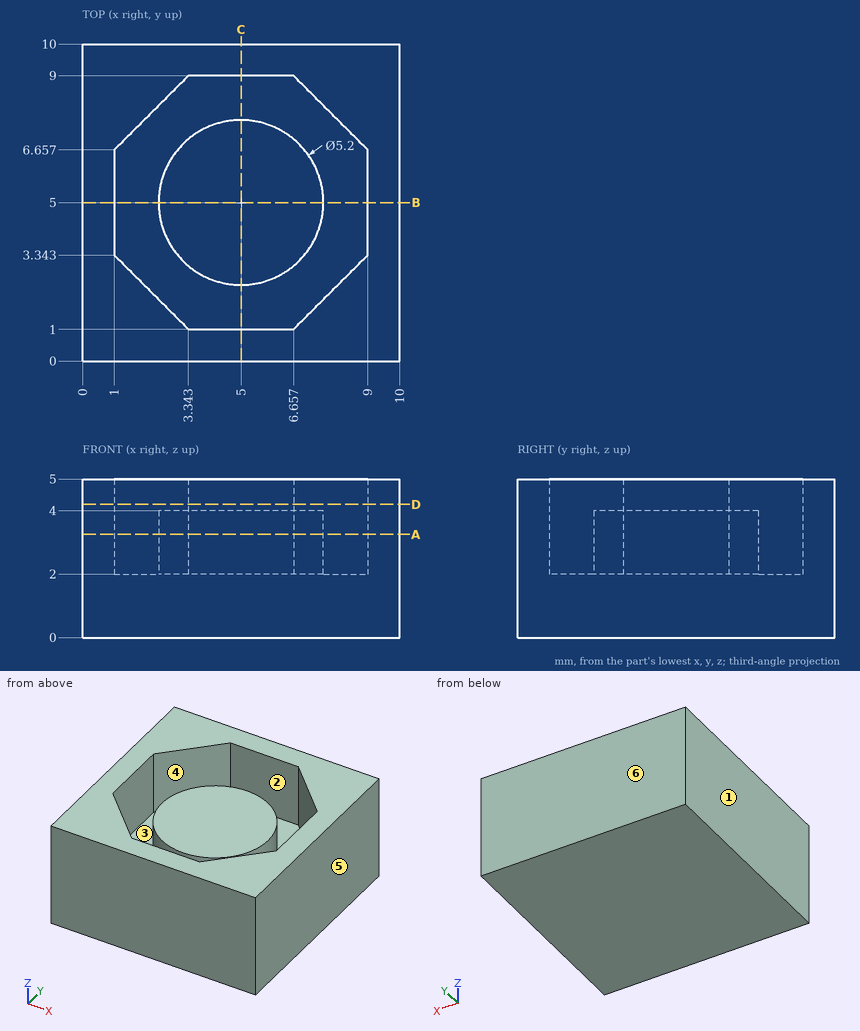
Answer from the drawing. Dimensions are ordinates in mm from the lowest x, y and z of the part. A direction names the side the tool comes from. Coordinates: 2 decimals unless noted, no trailing zeros. Loops run counter-clockwise (first coordinate to the right, second up) from the corner with the lowest first, then second, coordinate; pieces in that order, holes last. Notation, with made-up numbers: (87.5, 31) - (143.5, 31) arc R14 ccw to (143.5, 41) - close; hole circle Ø9 at (6, 13). An arc over 180 degrees is marked (long way). Use a Markdown table: item, result.
Item 1: Consider probe 1 along Y at (x, z) = (4, 2.1); probe 2 along Y at (x, z) = (6.25, 2.7); probe 3 along Y at (x, z) = (4, 4.4). Determine where each line is inside the solid, lowest interval first. Write a range as from..to.
Evaluation:
| item | result |
|---|---|
| probe 1 | y = 0..1, 2.6..7.4, 9..10 |
| probe 2 | y = 0..1, 2.72..7.28, 9..10 |
| probe 3 | y = 0..1, 9..10 |
Item 2: For the marked faces 1 and 2, determine the directions among +Z, -Z, +X, -X, +Y, -Y from which every point of the face is accessible in a straight line to the end or side of a thin tool.
Evaluation:
| item | result |
|---|---|
| face 1 | +Z, -Z, -X, +Y, -Y |
| face 2 | +Z |
Item 3: The mould has two halves that part along X. Classify the marked faces 3, 4, 5 and 6: +X half, -X half, draft (parallel to the pull), parting line (faces both ways), or undercut.
Evaluation:
| item | result |
|---|---|
| face 3 | undercut |
| face 4 | undercut |
| face 5 | +X half |
| face 6 | draft |
Item 4: Find section B-B, the plane y = 5. Determine the outline of the cut face in (x, z), and give its area (3 significant figures).
Evaluation:
| item | result |
|---|---|
| outline | (0, 0) - (10, 0) - (10, 5) - (9, 5) - (9, 2) - (7.6, 2) - (7.6, 4) - (2.4, 4) - (2.4, 2) - (1, 2) - (1, 5) - (0, 5) - close |
| area | 36.4 mm2 |
Item 5: Find section D-D, the plane z = 4.2. Determine the outline of the cut face in (x, y).
Evaluation:
| item | result |
|---|---|
| outline | (0, 0) - (10, 0) - (10, 10) - (0, 10) - close; hole (1, 3.34) - (3.34, 1) - (6.66, 1) - (9, 3.34) - (9, 6.66) - (6.66, 9) - (3.34, 9) - (1, 6.66) - close |
Item 6: Given pin 1 Ø2.5 at (x, y) = (3, 4) entering from +Z, flat-ended and moving along its own axis, determine where the tip first touches the part or whether it passes through.
Evaluation:
| item | result |
|---|---|
| pin 1 | stops at z = 4 |
Item 7: Find section A-A, the plane z = 3.25. Determine the outline of the cut face in (x, y), and give its area (3 significant figures).
Evaluation:
| item | result |
|---|---|
| outline | (0, 0) - (10, 0) - (10, 10) - (0, 10) - close; circle Ø5.2 at (5, 5); hole (1, 3.34) - (3.34, 1) - (6.66, 1) - (9, 3.34) - (9, 6.66) - (6.66, 9) - (3.34, 9) - (1, 6.66) - close |
| area | 68.2 mm2 |
